Read the model definition and answer for the solid it produces. Units are mm, in the model's axes. A direction names the side the tool comes from. Round coordinates to 2 decimals unless told otherwise and drop trailing zeros. Loops run counter-clockwise (first coordinate to the right, second up) from the corner with the lowest first, then second, coordinate; pieces in that order, holes last. Notation, with made-up numbers: M -18.75,77.5 L 22.25,77.5 A10 ccw 22.25,96.5 Z; hole C 68,-8 d4. An arc over 180 degrees is marked long. Answer as CSV lines item,"result".
```python
from build123d import *

# Parameters (mm, degrees)
F0_W = 23
F0_H = 6.5


with BuildPart() as f1:
    # F0 (on Top) → F1 (revolve)
    with BuildSketch(Plane.XY):
        with BuildLine():
            ThreePointArc((39.227544, -2.37903), (39.918853, -1.277694), (40.160403, 0))
            Line((40.160403, 0), (-62.651278, 0))
            Line((-62.651278, 0), (-62.651278, -6.5))
            Line((-62.651278, -6.5), (-62.651278, -10))
            Line((-62.651278, -10), (-49.651278, -10))
            ThreePointArc((-49.651278, -10), (-36.796792, -9.234882), (-24.424854, -12.806772))
            ThreePointArc((-24.424854, -12.806772), (8.879095, -17.705654), (38.9747, -2.625648))
            ThreePointArc((38.9747, -2.625648), (39.101317, -2.502538), (39.227544, -2.37903))
        make_face()
        with Locations((-74.151278, -3.25)):
            Rectangle(F0_W, F0_H)
    revolve(axis=Axis((-25.326952, 0, 0), (-1, 0, 0)))


solid = f1.part
```
1) A tool of negligible diameter and unlimited length cuts with its end or side. For faces 1 (the flat face through (-85.651, 0, 0)), 2 (the cylindrical face through (-56.06, 2.17, -9.76)), from which of +Z, -Z, +X, -X, +Y, -Y can it reach the whole face along a straight path? Write none if from no direction.
Evaluation:
face 1,"+Z, -Z, -X, +Y, -Y"
face 2,"-X"
2) Find section B-B, the plane x = -47.5. Give the vertices of the cut face in (y, z), then the cut area to 3 significant figures.
Evaluation:
outline,"C 0,0 d19.12"
area,"287 mm^2"
3) Each of these flat-tipped pins is pushed along its axis until it touches: P1, Ø8, axis at x = -34.5, y = -11, coming from the +Z side; P2, Ø2, axis at x = -15, y = -6.5, coming from the +Z side; P3, Ø12, axis at y = -10, z = 0.5, coming from the +X side. Where does it stop, or does it pass through?
Evaluation:
P1,"stops at z = 6.65"
P2,"stops at z = 15.52"
P3,"stops at x = 37.49"
4) Find section A-A, the plane x = -68. Give the vertices of the cut face in (y, z).
Evaluation:
outline,"C 0,0 d13"
5) Straight lines are drawn through the part: line 1 (Y direction, x = -52, z = 0.5); line 2 (Y direction, x = -44.5, z = -8); line 3 (X direction, y = -2, z = -6). For each, find the intervals that lie inside material, in ascending order.
Evaluation:
line 1,"y = -9.99 to 9.99"
line 2,"y = -4.47 to 4.47"
line 3,"x = -85.65 to 34.75"
